Autodesk Fusion 360 part; units mm, degrees
sketch "Sketch1" plane through (0, 0, 0) normal (0, 0, 1) x (1, 0, 0)
  line L0 (0, 0) -> (60, 0)
  line L1 (60, 0) -> (60, 19)
  line L2 (60, 19) -> (0, 19)
  line L3 (0, 19) -> (0, 0)
  line L4 (0, 19) -> (0, 34)
  line L5 (0, 34) -> (60, 34)
  line L6 (60, 34) -> (60, 19)
  line L7 (60, 19) -> (0, 19)
  line L8 (-2, 19) -> (-2, 36)
  line L9 (-2, 36) -> (62, 36)
  line L10 (62, 36) -> (62, 19)
  line L11 (62, -2) -> (62, 19)
  line L12 (-2, -2) -> (62, -2)
  line L13 (-2, 19) -> (-2, -2)
  dimension "d1" = 60
  dimension "d2" = 19
  dimension "d3" = 15
  dimension "d4" = 2
extrude "Extrude1" add sketch "Sketch1" along normal blind 50 contours L0 L1 L2 L3 L7
extrude "Extrude2" add sketch "Sketch1" against normal blind 5 contours L0 L1 L2 L3 L7 | L2 L4 L5 L6 L7 | L8 L9 L10 L11 L12 L13
sketch "Sketch2" plane through (0, 0, 0) normal (0, -1, 0) x (1, 0, 0)
  line L0 (0, 0) -> (60, 0)
  line L1 (60, 0) -> (60, 50)
  line L2 (60, 50) -> (0, 50)
  line L3 (0, 50) -> (0, 0)
  circle A0 centre (12, 40) radius 3
  circle A1 centre (48, 40) radius 3
  dimension "d11" = 6
  dimension "d12" = 6
  dimension "d13" = 12
  dimension "d14" = 10
  dimension "d15" = 10
  dimension "d16" = 12
hole "Hole1" at (12, 0, 40) direction (0, 1, 0) diameter 5.035 depth 19 tip angle 118
hole "Hole2" at (48, 0, 40) direction (0, 1, 0) diameter 5.035 depth 19 tip angle 118
fillet "Fillet1" radius 2 4 edges at (62, 36, -2.5) (-2, 36, -2.5) (62, -2, -2.5) (-2, -2, -2.5)
fillet "Fillet2" radius 1 4 edges at (0, 0, 25) (0, 19, 25) (60, 0, 25) (60, 19, 25)
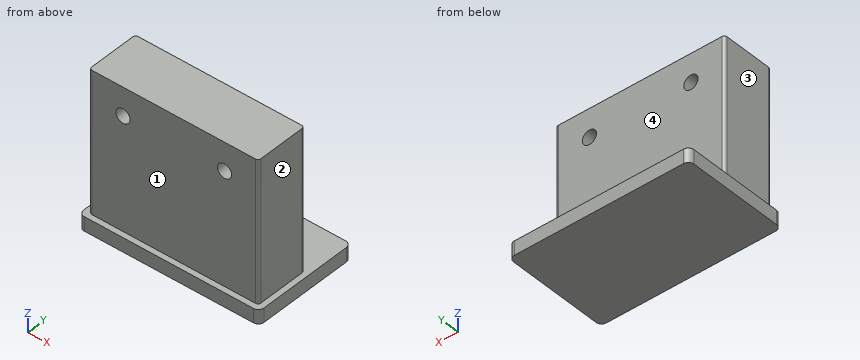
Work out the finished part from the listing and answer in its coordinate system (mm). Face numbers are marked on the shaded views. A direction names the side the tool comes from. Coordinates: 2 decimals unless noted, no trailing zeros. Write each loop counter-clockwise with the first axis right and the second up, starting at its lowest first coordinate (ties: lowest second). Pieces come first, ordered by that corner, then holes.
1. Flat-ended cylindrical pins translate along their axes: pin 1 (25 mm diameter, centred on x = 24, z = 36, fed in from +Y); pin 2 (6.5 mm diameter, centred on x = 12, z = 40, fed in from -Y); pin 3 (8.5 mm diameter, centred on y = 7, z = 24.5, fed in from -X). Find the tip coordinate at first contact, or state that the pin passes through.
Results list:
pin 1: stops at y = 19
pin 2: stops at y = 0
pin 3: stops at x = 0
2. The part is cut by section C-C, the plane y = 5. Write down the section's boundary in (x, z) (1 decimal).
Results list:
outline: (-2, -5) - (62, -5) - (62, 0) - (60, 0) - (60, 50) - (0, 50) - (0, 0) - (-2, 0) - close; hole circle Ø5 at (12, 40); hole circle Ø5 at (48, 40)
3. For the marked faces 1, 2, 3 and 4, determine the directions among +Z, -Z, +X, -X, +Y, -Y from which every point of the face is accessible in a straight line to the end or side of a thin tool.
Results list:
face 1: +Z, +X, -X, -Y
face 2: +Z, +X, +Y, -Y
face 3: +Z, -X, +Y, -Y
face 4: +Z, +X, -X, +Y
4. Consider line 1 along X through (y, z) = (9.25, 40); line 2 along Z through (x, y) = (48, 13); line 3 along Y through (x, z) = (10, 29.5). Determine where each line is inside the solid, lowest interval first.
Results list:
line 1: x = 0 to 9.48, 14.52 to 45.48, 50.52 to 60
line 2: z = -5 to 37.48, 42.52 to 50
line 3: y = 0 to 19
5. The part is cut by section A-A, the plane x = 12. Write down the section's boundary in (y, z), and give its area (3 significant figures).
Results list:
outline: (-2, -5) - (36, -5) - (36, 0) - (19, 0) - (19, 37.48) - (0, 37.48) - (0, 0) - (-2, 0) - close; (0, 42.52) - (19, 42.52) - (19, 50) - (0, 50) - close
area: 1,040 mm2
6. The part is cut by section B-B, the plane z = 40. Write down the section's boundary in (x, y), and give its area (3 significant figures).
Results list:
outline: (0, 1) arc R1 ccw to (1, 0) - (9.48, 0) - (9.48, 19) - (1, 19) arc R1 ccw to (0, 18) - close; (14.52, 0) - (45.48, 0) - (45.48, 19) - (14.52, 19) - close; (50.52, 0) - (59, 0) arc R1 ccw to (60, 1) - (60, 18) arc R1 ccw to (59, 19) - (50.52, 19) - close
area: 948 mm2
7. The part is cut by section D-D, the plane x = 5. Write down the section's boundary in (y, z).
Results list:
outline: (-2, -5) - (36, -5) - (36, 0) - (19, 0) - (19, 50) - (0, 50) - (0, 0) - (-2, 0) - close
